For this review, take the finished solid that the model builds, in its own axes (mm). Coordinates: 2 decimals unless noted, no trailing zeros. Write each loop counter-clockwise with the first axis right and the second up, starting at its lowest first coordinate (ties: lowest second). Pieces come first, ordered by that corner, then holes.
```python
from build123d import *

# Parameters (mm, degrees)
SKETCH1_R           = 28
SKETCH1_R_2         = 15
BOSS_EXTRUDE1_DEPTH = 106
BOSS_EXTRUDE3_DEPTH = 53
CUT_EXTRUDE1_DEPTH  = 128
CUT_EXTRUDE2_DEPTH  = 123


with BuildPart() as part:
    # Sketch1 → Boss-Extrude1 (new body)
    with BuildSketch(Plane.XY):
        Circle(SKETCH1_R)
        Circle(SKETCH1_R_2, mode=Mode.SUBTRACT)
    extrude(amount=BOSS_EXTRUDE1_DEPTH)

    # Sketch2 → Boss-Extrude3 (add, symmetric)
    with BuildSketch(Plane(origin=(0, 0, 0), x_dir=(1, 0, 0), z_dir=(0, 1, 0))):
        with BuildLine():
            ThreePointArc((-28, -26.846606339), (-66, -53), (-28, -79.153393661))
            Line((-28, -79.153393661), (-28, -64.180339887))
            ThreePointArc((-28, -64.180339887), (-53, -53), (-28, -41.819660113))
            Line((-28, -41.819660113), (-28, -26.846606339))
        make_face()
        with BuildLine():
            Line((-28, -64.180339887), (-28, -79.153393661))
            ThreePointArc((-28, -79.153393661), (-14.934874811, -68.874507866), (-10, -53))
            ThreePointArc((-10, -53), (-14.934874811, -37.125492134), (-28, -26.846606339))
            Line((-28, -26.846606339), (-28, -41.819660113))
            ThreePointArc((-28, -41.819660113), (-24.306936062, -46.876275643), (-23, -53))
            ThreePointArc((-23, -53), (-24.306936062, -59.123724357), (-28, -64.180339887))
        make_face()
    extrude(amount=BOSS_EXTRUDE3_DEPTH, both=True)

    # Sketch3 → Cut-Extrude1 (cut, symmetric)
    with BuildSketch(Plane.XY):
        with BuildLine():
            Line((-10, 11.180339887), (-10, -11.180339887))
            ThreePointArc((-10, -11.180339887), (-15, 0), (-10, 11.180339887))
        make_face()
    extrude(amount=CUT_EXTRUDE1_DEPTH, both=True, mode=Mode.SUBTRACT)

    # Sketch4 → Cut-Extrude2 (cut, symmetric)
    with BuildSketch(Plane(origin=(0, 0, 0), x_dir=(1, 0, 0), z_dir=(0, 1, 0))):
        with BuildLine():
            Line((-28, -64.180339887), (-28, -41.819660113))
            ThreePointArc((-28, -41.819660113), (-23, -53), (-28, -64.180339887))
        make_face()
    extrude(amount=CUT_EXTRUDE2_DEPTH, both=True, mode=Mode.SUBTRACT)


solid = part.part
```
1) Consider section C-C (y = 13.5). Give the boundary of the cut face in (x, z).
2) Consider section A-A (x = 0). Give the boundary of the cut face in (y, z), then the cut area to 3 significant figures.
3) Clearance check with flat-ended pins moving along their axes: P1, Ø4, axis at x = -25, y = -23.5, coming from the +Z side; P2, Ø2, axis at x = -13, z = 89, coming from the -Y side; P3, Ø3, axis at x = -14, y = 37.5, coming from the -Z side. State where each tip first meets the part, or that it passes through.
4) For L1, parallel to X at y = -0.5, z = 53; L2, parallel to X at y = 12.5, z = 53; L3, parallel to X at y = 23, z = 53, list the stretches that pass through material, from the lowest coordinate up.
5) Consider section B-B (z = 44.5). Give the boundary of the cut face in (x, y).
6) Consider section D-D (y = -45.5). Give the boundary of the cut face in (x, z).
7) The part is to be moulded in two halves that separate along X. For faces 1 (the face through (26.707, 8.41, 52.258)), 2 (the face through (12, -12, 0)), say which applies: pulls with the +X half, pulls with the -X half, needs draft (parallel to the pull), parting line crosses it, or undercut.
Results:
1. outline: (-24.53, 0) - (-6.54, 0) - (-6.54, 106) - (-24.53, 106) - (-24.53, 77.55) arc R28 ccw (long way) to (-24.53, 28.45) - close; (6.54, 0) - (24.53, 0) - (24.53, 106) - (6.54, 106) - close; hole circle Ø30 at (-38, 53)
2. outline: (-28, 0) - (-15, 0) - (-15, 106) - (-28, 106) - close; (15, 0) - (28, 0) - (28, 106) - (15, 106) - close
2. area: 2,760 mm2
3. P1: stops at z = 78.75
3. P2: stops at y = -25.3
3. P3: stops at z = 36.33
4. L1: x = -66 to -53, -23 to -14.99, 14.99 to 28
4. L2: x = -66 to -53, -23 to -8.29, 8.29 to 25.05
4. L3: x = -66 to -53, -23 to 15.97
5. outline: (-64.68, -53) - (-50.36, -53) - (-50.36, 53) - (-64.68, 53) - close; (-25.64, -53) - (-11.32, -53) - (-11.32, -25.61) arc R28 ccw (long way) to (-11.32, 25.61) - (-11.32, 53) - (-25.64, 53) - close; hole circle Ø30 at (0, 0)
6. outline: circle Ø56 at (-38, 53); hole circle Ø30 at (-38, 53)
7. face 1: undercut
7. face 2: needs draft
